Read the model definition and answer for the solid it produces. Units are mm, in the model's axes. Face numbers are marked on the shaded views. A direction names the side the tool comes from. Give positions to 0.01 mm unless a question says otherwise; leave off trailing zeros. Write each loop counter-clockwise with the first axis right and the second up, starting at its lowest first coordinate (ties: lowest second). Pieces come first, ordered by that corner, then holes. Notation, with made-up numbers: (64.5, 51) -> (100.5, 51) arc R20 ccw to (100.5, 86) -> close; hole circle Ø9 at (-6, 4.25). An arc over 180 degrees is marked (long way). Use a Markdown table: item, result.
from build123d import *

# Parameters (mm, degrees)
F1_DEPTH     = 50
F2_W         = 20
F2_H         = 100
F3_DEPTH     = 40
F4_R         = 2.5
F5_DEPTH     = 10
F6_W         = 90
F6_H         = 90
F7_DEPTH     = 20
F8_R         = 5
F9_DEPTH     = 20
F10_R        = 1.5
F11_DEPTH    = 40
F12_SIZE     = 3
F13_T1_DEPTH = 30
F13_T3_DEPTH = 30
F13_T5_DEPTH = 30


# Not quite as in the source:
# - a fillet or chamfer that OpenCascade refuses, or shapes differently, is made with other operations: its cross-section is extruded or revolved along the edge and cut away or added


with BuildPart() as f1:
    # F0 (on Top) → F1 (new body)
    with BuildSketch(Plane.XY):
        Polygon((-50, -50), (50, -50), (70, -50), (70, 50), (50, 50), (-50, 50), align=None)
    extrude(amount=F1_DEPTH)

    # F2 (on face) → F3 (cut)
    with BuildSketch(Plane.XY.offset(50)):
        with Locations((60, 0)):
            Rectangle(F2_W, F2_H)
    extrude(amount=-F3_DEPTH, mode=Mode.SUBTRACT)

    # F4 (on face) → F5 (cut, through all)
    with BuildSketch(Plane.XY.offset(10)):
        with BuildLine():
            Line((50, -40), (50, -50))
            Line((50, -50), (70, -50))
            Line((70, -50), (70, -35))
            Line((70, -35), (55, -35))
            ThreePointArc((55, -35), (51.4644660941, -36.4644660941), (50, -40))
        make_face()
        with Locations((60, -25)):
            Circle(F4_R)
        with Locations((60, 25)):
            Circle(F4_R)
        with BuildLine():
            ThreePointArc((50, 40), (51.4644660941, 36.4644660941), (55, 35))
            Line((55, 35), (70, 35))
            Line((70, 35), (70, 50))
            Line((70, 50), (50, 50))
            Line((50, 50), (50, 40))
        make_face()
    extrude(amount=-F5_DEPTH, mode=Mode.SUBTRACT)

    # F6 (on face) → F7 (cut)
    with BuildSketch(Plane.XY.offset(50)):
        Rectangle(F6_W, F6_H)
    extrude(amount=-F7_DEPTH, mode=Mode.SUBTRACT)

    # F8 (on face) → F9 (cut)
    with BuildSketch(Plane.XY.offset(30)):
        with Locations((-32.5000025332, 32.5000174344)):
            Circle(F8_R)
        Polygon((-45.0000017881, 20.0000017881), (-45.0000017881, -20.0000017881), (-20.0000017881, -20.0000017881), (-20.0000017881, -45.0000017881), (20.0000017881, -45.0000017881), (20.0000017881, -20.0000017881), (45.0000017881, -20.0000017881), (45.0000017881, 20.0000017881), (20.0000017881, 20.0000017881), (20.0000017881, 45.0000017881), (-20.0000017881, 45.0000017881), (-20.0000017881, 20.0000017881), align=None)
        with Locations((-32.5000025332, -32.5000174344)):
            Circle(F8_R)
        with Locations((32.5000025332, 32.5000174344)):
            Circle(F8_R)
        with Locations((32.5000025332, -32.5000174344)):
            Circle(F8_R)
    extrude(amount=-F9_DEPTH, mode=Mode.SUBTRACT)

    # F10 (on face) → F11 (cut)
    with BuildSketch(Plane.XY.offset(50)):
        with Locations((-46.5, 46.5)):
            Circle(F10_R)
        with Locations((-46.5, -46.5)):
            Circle(F10_R)
        with Locations((46.5, 46.5)):
            Circle(F10_R)
        with Locations((46.5, -46.5)):
            Circle(F10_R)
    extrude(amount=-F11_DEPTH, mode=Mode.SUBTRACT)

    # F12
    f12_edges = [f1.edges().sort_by_distance(p)[0] for p in [
        (70, -35, 5),
        (70, 35, 5),
        (50, -50, 25),
        (-50, -50, 25),
        (50, 50, 25),
        (-50, 50, 25),
    ]]
    chamfer(f12_edges, length=F12_SIZE)

    # F13: fillet of radius 4 on 16 edges, made by hand

    # F13_s2 → F13_t1 (join)
    with BuildSketch(Plane.XY.offset(20)):
        with BuildLine():
            ThreePointArc((-45, 41), (-43.8284271247, 43.8284271247), (-41, 45))
            Line((-41, 45), (-45, 45))
            Line((-45, 45), (-45, 41))
        make_face()
        with BuildLine():
            ThreePointArc((45, 41), (43.8284271247, 43.8284271247), (41, 45))
            Line((41, 45), (45, 45))
            Line((45, 45), (45, 41))
        make_face()
        with BuildLine():
            ThreePointArc((41, -45), (43.8284271247, -43.8284271247), (45, -41))
            Line((45, -41), (45, -45))
            Line((45, -45), (41, -45))
        make_face()
        with BuildLine():
            ThreePointArc((-41, -45), (-43.8284271247, -43.8284271247), (-45, -41))
            Line((-45, -41), (-45, -45))
            Line((-45, -45), (-41, -45))
        make_face()
    extrude(amount=F13_T1_DEPTH)

    # F13_s4 → F13_t3 (join)
    with BuildSketch(Plane.XY):
        with BuildLine():
            ThreePointArc((-41.0000017881, 20.0000017881), (-43.8284289129, 18.8284289129), (-45.0000017881, 16.0000017881))
            Line((-45.0000017881, 16.0000017881), (-45.0000017881, 20.0000017881))
            Line((-45.0000017881, 20.0000017881), (-41.0000017881, 20.0000017881))
        make_face()
        with BuildLine():
            ThreePointArc((-20.0000017881, 41.0000017881), (-18.8284289129, 43.8284289129), (-16.0000017881, 45.0000017881))
            Line((-16.0000017881, 45.0000017881), (-20.0000017881, 45.0000017881))
            Line((-20.0000017881, 45.0000017881), (-20.0000017881, 41.0000017881))
        make_face()
        with BuildLine():
            ThreePointArc((20.0000017881, 41.0000017881), (18.8284289129, 43.8284289129), (16.0000017881, 45.0000017881))
            Line((16.0000017881, 45.0000017881), (20.0000017881, 45.0000017881))
            Line((20.0000017881, 45.0000017881), (20.0000017881, 41.0000017881))
        make_face()
        with BuildLine():
            ThreePointArc((41.0000017881, 20.0000017881), (43.8284289129, 18.8284289129), (45.0000017881, 16.0000017881))
            Line((45.0000017881, 16.0000017881), (45.0000017881, 20.0000017881))
            Line((45.0000017881, 20.0000017881), (41.0000017881, 20.0000017881))
        make_face()
        with BuildLine():
            ThreePointArc((-41.0000017881, -20.0000017881), (-43.8284289129, -18.8284289129), (-45.0000017881, -16.0000017881))
            Line((-45.0000017881, -16.0000017881), (-45.0000017881, -20.0000017881))
            Line((-45.0000017881, -20.0000017881), (-41.0000017881, -20.0000017881))
        make_face()
        with BuildLine():
            ThreePointArc((-20.0000017881, -41.0000017881), (-18.8284289129, -43.8284289129), (-16.0000017881, -45.0000017881))
            Line((-16.0000017881, -45.0000017881), (-20.0000017881, -45.0000017881))
            Line((-20.0000017881, -45.0000017881), (-20.0000017881, -41.0000017881))
        make_face()
        with BuildLine():
            ThreePointArc((20.0000017881, -41.0000017881), (18.8284289129, -43.8284289129), (16.0000017881, -45.0000017881))
            Line((16.0000017881, -45.0000017881), (20.0000017881, -45.0000017881))
            Line((20.0000017881, -45.0000017881), (20.0000017881, -41.0000017881))
        make_face()
        with BuildLine():
            ThreePointArc((41.0000017881, -20.0000017881), (43.8284289129, -18.8284289129), (45.0000017881, -16.0000017881))
            Line((45.0000017881, -16.0000017881), (45.0000017881, -20.0000017881))
            Line((45.0000017881, -20.0000017881), (41.0000017881, -20.0000017881))
        make_face()
    extrude(amount=F13_T3_DEPTH)

    # F13_s6 → F13_t5 (cut)
    with BuildSketch(Plane.XY.offset(10)):
        with BuildLine():
            ThreePointArc((-20.0000017881, 24.0000017881), (-21.1715746634, 21.1715746634), (-24.0000017881, 20.0000017881))
            Line((-24.0000017881, 20.0000017881), (-20.0000017881, 20.0000017881))
            Line((-20.0000017881, 20.0000017881), (-20.0000017881, 24.0000017881))
        make_face()
        with BuildLine():
            ThreePointArc((24.0000017881, 20.0000017881), (21.1715746634, 21.1715746634), (20.0000017881, 24.0000017881))
            Line((20.0000017881, 24.0000017881), (20.0000017881, 20.0000017881))
            Line((20.0000017881, 20.0000017881), (24.0000017881, 20.0000017881))
        make_face()
        with BuildLine():
            ThreePointArc((-24.0000017881, -20.0000017881), (-21.1715746634, -21.1715746634), (-20.0000017881, -24.0000017881))
            Line((-20.0000017881, -24.0000017881), (-20.0000017881, -20.0000017881))
            Line((-20.0000017881, -20.0000017881), (-24.0000017881, -20.0000017881))
        make_face()
        with BuildLine():
            ThreePointArc((24.0000017881, -20.0000017881), (21.1715746634, -21.1715746634), (20.0000017881, -24.0000017881))
            Line((20.0000017881, -24.0000017881), (20.0000017881, -20.0000017881))
            Line((20.0000017881, -20.0000017881), (24.0000017881, -20.0000017881))
        make_face()
    extrude(amount=F13_T5_DEPTH, mode=Mode.SUBTRACT)


solid = f1.part
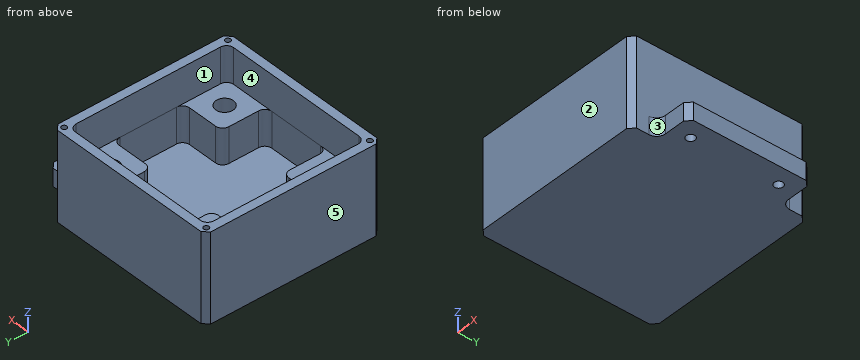
Item 1: Each of these flat-tipped pins is pushed along its axis until it touches: P1, Ø0.9, axis at x = -46.5, y = 46, coming from the +Z side; P2, Ø4, axis at y = 28, z = 41, coming from the +X side; P3, Ø11.5, axis at x = -32.5, y = -32.5, coming from the +Z side. Where does it stop, or does it pass through?
Return value:
| item | result |
|---|---|
| P1 | z = 10 |
| P2 | x = 50 |
| P3 | z = 30 |
Item 2: Straight lines are drawn through the part: line 1 along Y through (x, z) = (60, 4); line 2 along Y through (x, z) = (32, 26); line 3 along X through (y, z) = (-38.5, 15). For each, find the intervals that lie inside material, in ascending order. Write a range as [from, to].
Return value:
| item | result |
|---|---|
| line 1 | [-35, -27.5], [-22.5, 22.5], [27.5, 35] |
| line 2 | [-50, -37.47], [-27.53, -20], [20, 27.53], [37.47, 50] |
| line 3 | [-50, -20], [20, 50] |
Item 3: A cutting plane is placed at A-A (x = 60). Give the vertices of the cut face in (y, z), then the cut area to 3 significant figures.
Return value:
| item | result |
|---|---|
| outline | (-35, 0) -> (-27.5, 0) -> (-27.5, 10) -> (-35, 10) -> close; (-22.5, 0) -> (22.5, 0) -> (22.5, 10) -> (-22.5, 10) -> close; (27.5, 0) -> (35, 0) -> (35, 10) -> (27.5, 10) -> close |
| area | 600 mm^2 |
Item 4: A cutting plane is placed at B-B (z = 37). Give the vertices of the cut face in (x, y), then the cut area to 3 significant figures.
Return value:
| item | result |
|---|---|
| outline | (-50, -47) -> (-47, -50) -> (47, -50) -> (50, -47) -> (50, 47) -> (47, 50) -> (-47, 50) -> (-50, 47) -> close; hole circle Ø3 at (-46.5, -46.5); hole circle Ø3 at (-46.5, 46.5); hole (-45, -41) arc R4 ccw to (-41, -45) -> (41, -45) arc R4 ccw to (45, -41) -> (45, 41) arc R4 ccw to (41, 45) -> (-41, 45) arc R4 ccw to (-45, 41) -> close; hole circle Ø3 at (46.5, -46.5); hole circle Ø3 at (46.5, 46.5) |
| area | 1,870 mm^2 |
Item 5: For a pull along Y with two mould halves and no side action, classify the marked faces 3, 4 and 5 as +Y half, -Y half, draft (parallel to the pull), parting line (faces both ways), or undercut.
Return value:
| item | result |
|---|---|
| face 3 | -Y half |
| face 4 | undercut |
| face 5 | draft |
Item 6: A tool of negligible diameter and unlimited length cuts with its end or side. For the marked faces 1 and 2, from which of +Z, -Z, +X, -X, +Y, -Y can it reach the whole face along a straight path? Write none if from no direction.
Return value:
| item | result |
|---|---|
| face 1 | +Z |
| face 2 | +Z, -Z, +X, -X, -Y |
